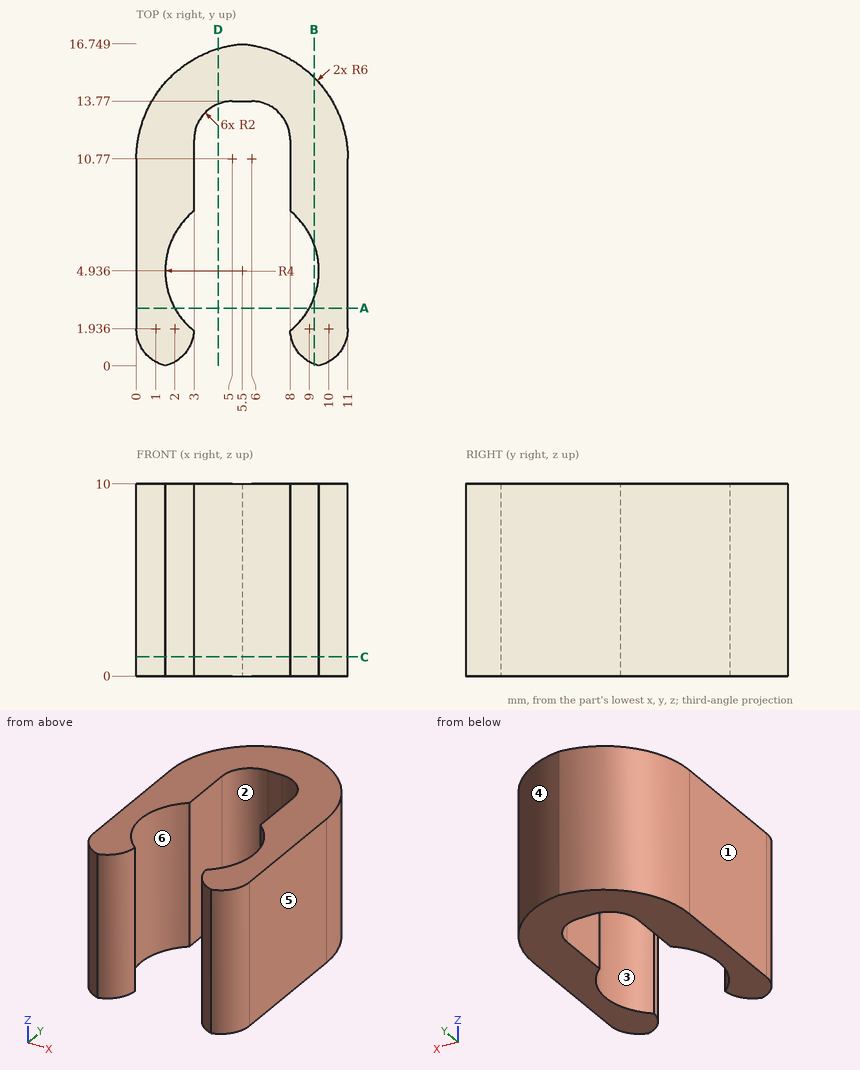
For this review, use the dimensioned drawing (mm, ordinates from the lowest corner) and the shaded views. A direction names the side the tool comes from. Coordinates: 2 decimals unless noted, no trailing zeros. Loops run counter-clockwise (first coordinate to the right, second up) from the corner with the lowest first, then second, coordinate; pieces in that order, holes last. Notation, with made-up numbers: (77, 87) -> (118, 87) arc R8 ccw to (118, 97) -> close; hole circle Ø3 at (2, 7). An arc over 180 degrees is marked (long way). Return JSON: item names as keys, results as strings. Group by question number.
(1) For pin 1 Ø1 at (x, z) = (6, 9) entering from -Y; pin 2 Ø0.8 at (x, z) = (5.5, 6.5) entering from -Y, all flat-tipped, find the tip position at first contact; note any pin that passes through.
(2) To check wall thickness, follow L1, parallel to X at y = 5, z = 2; L2, parallel to Y at x = 2.5, z = 6.5 (1 decimal); L3, parallel to X at y = 7.75, z = 8.25 (1 decimal). State the ranges of each line that lie inside material, in increasing order.
(3) Mouldability with a two-part tool opening along Y and no side actions: class the marked faces 3, 4, 5 and 6 as pulls with the +Y half, pulls with the -Y half, needs draft (parallel to the pull), parting line crosses it, or undercut.
(4) Consider section B-B, the plane x = 9.25. Give the boundary of the cut face in (y, z) (1 decimal), plus the area to 3 significant figures.
(5) Consider section A-A, the plane y = 3. Give the boundary of the cut face in (x, z), plus the area to 3 significant figures.
(6) Consider section C-C, the plane z = 1. Give the boundary of the cut face in (x, y).
(7) Tool access review of the marked faces 1 and 2: name each direction out of +Z, -Z, +X, -X, +Y, -Y from which nothing blocks a thin tool from reaching the whole face with its end or side.
(8) Consider section D-D, the plane x = 4.25. Give the boundary of the cut face in (y, z).
Results below:
{
 "1": {"pin 1": "stops at y = 13.71", "pin 2": "stops at y = 13.77"},
 "2": {"L1": "x = 0 to 1.5, 9.5 to 11", "L2": "y = 0.6 to 2.3, 7.6 to 15.6", "L3": "x = 0 to 2.7, 8.3 to 11"},
 "3": {"face 3": "undercut", "face 4": "pulls with the +Y half", "face 5": "needs draft", "face 6": "undercut"},
 "4": {"outline": "(0.1, 0) -> (3.5, 0) -> (3.5, 10) -> (0.1, 10) -> close; (6.3, 0) -> (15, 0) -> (15, 10) -> (6.3, 10) -> close", "area": "121 mm2"},
 "5": {"outline": "(0, 0) -> (2, 0) -> (2, 10) -> (0, 10) -> close; (9, 0) -> (11, 0) -> (11, 10) -> (9, 10) -> close", "area": "40.0 mm2"},
 "6": {"outline": "(0, 1.94) arc R2 ccw to (1.5, 0) arc R2 ccw to (3, 1.82) arc R4 cw to (3, 8.06) -> (3, 11.77) arc R2 cw to (5, 13.77) -> (6, 13.77) arc R2 cw to (8, 11.77) -> (8, 8.06) arc R4 cw to (8, 1.82) arc R2 ccw to (9.5, 0) arc R2 ccw to (11, 1.94) -> (11, 10.77) arc R6 ccw to (5.5, 16.75) arc R6 ccw to (0, 10.77) -> close"},
 "7": {"face 1": "+Z, -Z, -X, +Y, -Y", "face 2": "+Z, -Z, -Y"},
 "8": {"outline": "(13.62, 0) -> (16.51, 0) -> (16.51, 10) -> (13.62, 10) -> close"}
}
